Design review of the part built by this model. Coordinates are the model's own, in mm. A direction names the side the tool comes from. Round coordinates to 2 decimals unless told otherwise and drop trailing zeros. Write each loop counter-clockwise with the first axis right and the second up, starting at its lowest first coordinate (ties: lowest second). Pieces come first, ordered by that corner, then holes. Notation, with made-up numbers: (62.5, 17.5) -> (81.5, 17.5) arc R12 ccw to (81.5, 37.5) -> close; hole circle Ø3 at (55, 2). An arc over 180 degrees is marked (long way). Write item = value, one per line. Start each with the question number.
Item 1: Add section D-D, the plane z = -169.5. State the section outline as (x, y) points.
Item 2: For pin 1 Ø4 at (x, y) = (-271, -118.5) entering from -Z; pin 2 Ø6 at (y, z) = (-128.5, -93.5) entering from +X, all flat-tipped, find the tip position at first contact; note any pin that passes through.
Item 3: Add section A-A, the plane z = -117.5. State the section outline as (x, y) points.
Item 4: Mouldability with a two-part tool opening along X and no side actions: class faces 3 (the flat face through (-228, 3, -100)), 4 (the flat face through (-228, 3, -80)), 5 (the flat face through (0, -3, -128)) as released by +X, released by -X, zero draft, split by the parting line, or undercut.
Item 5: Add section B-B, the plane y = -83.5. State the section outline as (x, z) points, then the cut area to 3 significant figures.
Item 6: Machinability: for faces 1 (the flat face through (-430, 2, -138)), 2 (the cylindrical face through (-440.14, 2.93, -199.98)), which of the approach directions +Z, -Z, +X, -X, +Y, -Y give a long, thin tool a straight path to every point of the face, cutting with its end or side? Answer none if there is none.
Item 7: To check wall thickness, follow L1, parallel to X at y = -42, z = -164; L2, parallel to Z at x = -276, y = 136. State the ranges of each line that lie inside material, in increasing order.
Item 8: Add section C-C, the plane x = -422. State the section outline as (y, z) points, then the cut area to 3 significant figures.
from build123d import *

# Parameters (mm, degrees)
F1_DEPTH = 20
F2_W     = 450
F2_H     = 450
F3_DEPTH = 20
F5_DEPTH = 20


with BuildPart() as f1:
    # F0 (on Right) → F1 (new body)
    with BuildSketch(Plane.YZ):
        with BuildLine():
            Line((173.2050807569, -100), (-173.2050807569, -100))
            ThreePointArc((-173.2050807569, -100), (0, -200), (173.2050807569, -100))
        make_face()
    extrude(amount=-F1_DEPTH)

    # F2 (on face) → F3 (join)
    with BuildSketch(Plane.XY.offset(-100)):
        with Locations((-225, 0)):
            Rectangle(F2_W, F2_H)
        Polygon((0, 225), (-450, 225), (-450, -225), (0, -225), (0, -173.2050807569), (-20, -173.2050807569), (-20, 173.2050807569), (0, 173.2050807569), align=None)
    extrude(amount=F3_DEPTH)

    # F4 (on face) → F5 (join)
    with BuildSketch(Plane(origin=(-450, 0, 0), x_dir=(0, -1, 0), z_dir=(-1, 0, 0))):
        with BuildLine():
            Line((173.2050807569, -100), (-173.2050807569, -100))
            ThreePointArc((-173.2050807569, -100), (0, -200), (173.2050807569, -100))
        make_face()
    extrude(amount=-F5_DEPTH)


solid = f1.part
Result set:
q1.outline = (-450, -106.16) -> (-430, -106.16) -> (-430, 106.16) -> (-450, 106.16) -> close; (-20, -106.16) -> (0, -106.16) -> (0, 106.16) -> (-20, 106.16) -> close
q2.pin_1 = -100
q2.pin_2 = 0
q3.outline = (-450, -161.84) -> (-430, -161.84) -> (-430, 161.84) -> (-450, 161.84) -> close; (-20, -161.84) -> (0, -161.84) -> (0, 161.84) -> (-20, 161.84) -> close
q4.face_3 = undercut
q4.face_4 = zero draft
q4.face_5 = released by +X
q5.outline = (-450, -181.74) -> (-430, -181.74) -> (-430, -100) -> (-20, -100) -> (-20, -181.74) -> (0, -181.74) -> (0, -80) -> (-450, -80) -> close
q5.area = 12,300 mm²
q6.face_1 = -Z, +Y, -Y
q6.face_2 = -Z, +X, -X
q7.L1 = -450 to -430, -20 to 0
q7.L2 = -100 to -80
q8.outline = (-225, -100) -> (225, -100) -> (225, -80) -> (-225, -80) -> close
q8.area = 9,000 mm²
